Autodesk Inventor part; units mm, degrees
ref_plane "YZ Plane" through (0, 0, 0) normal (1, 0, 0) x (0, 1, 0)
ref_plane "XZ Plane" through (0, 0, 0) normal (0, 1, 0) x (-1, 0, 0)
ref_plane "XY Plane" through (0, 0, 0) normal (0, 0, 1) x (1, 0, 0)
sketch "スケッチ1" plane through (0, 0, 0) normal (1, 0, 0) x (0, 1, 0)
  circle A0 centre (0, 0) radius 17.5
  dimension "d0" = 35
extrude "押し出し1" add sketch "スケッチ1" along normal blind 3
sketch "スケッチ2" plane through (3, 0, 0) normal (1, 0, 0) x (0, 0, -1)
  circle A0 centre (0, 0) radius 13.5
  point P0 (13.5, 0)
  point P1 (6.75, 11.6913)
  point P2 (-6.75, 11.6913)
  point P3 (-13.5, 0)
  point P4 (-6.75, -11.6913)
  point P5 (6.75, -11.6913)
  dimension "d3" = 27
  dimension "d6" = 360
hole "穴1" at (3, 0, -13.5) at (3, 11.6913, -6.75) at (3, 11.6913, 6.75) at (3, 0, 13.5) at (3, -11.6913, 6.75) at (3, -11.6913, -6.75) direction (-1, 0, 0) diameter 3.2 end through all
sketch "スケッチ4" plane through (3, 0, 0) normal (1, 0, 0) x (0, 0, -1)
  circle A0 centre (0, 0) radius 20
  circle A1 centre (0, -20) radius 5
  circle A2 centre (0, 20) radius 5
  circle A3 centre (13.5, 0) radius 1.6
  circle A4 centre (-13.5, 0) radius 1.6
  line L0 (-24.9861, -3.2077) -> (0.509, 28.6357)
  line L1 (1.3172, 26.3548) -> (24.4586, -2.5487)
  line L2 (-28.3137, 7.3638) -> (1.2125, -29.5144)
  line L3 (-0.4955, -28.6189) -> (23.5579, 1.4238)
  circle A5 centre (0, 0) radius 17.5
  point P0 (-3.9031, 23.125)
  point P1 (-13.6609, 10.9375)
  point P2 (-13.6609, -10.9375)
  point P3 (-3.9031, -23.125)
  point P4 (3.9031, -23.125)
  point P5 (13.6609, -10.9375)
  point P6 (13.6609, 10.9375)
  point P7 (3.9031, 23.125)
  dimension "d22" = 40
  dimension "d23" = 10
  dimension "d24" = 10
  dimension "d25" = 13.5
  dimension "d26" = 13.5
extrude "押し出し2" add sketch "スケッチ4" against normal blind 2 contours L1 A5 A2 A0 | A0 A2 L1 | A5 A1 A2 | L3 A1 A0 | A0 A1 A5 L3 | A2 A5 A0 | A0 A2 | A2 A5 | A1 A0 | A0 A1 A5 | A5 A1 | A2 A5 L0 A0 | A0 L0 A2 | A1 L2 A0 | A0 L2 A5 A1
sketch "スケッチ5" plane through (0, 0, 0) normal (-1, 0, 0) x (0, 0, 1)
  circle A0 centre (6.75, -11.6913) radius 1.6
  circle A1 centre (-6.75, -11.6913) radius 1.6
  circle A2 centre (-6.75, 11.6913) radius 1.6
  circle A3 centre (6.75, 11.6913) radius 1.6
  arc A4 (3.9031, 23.125) -> (-3.9031, 23.125) centre (0, 20) ccw
  arc A5 (-3.9031, -23.125) -> (3.9031, -23.125) centre (0, -20) ccw
  point P0 (0, 0)
hole "穴2" at (0, -11.6913, 6.75) at (0, -11.6913, -6.75) at (0, 11.6913, -6.75) at (0, 11.6913, 6.75) at (0, 20, 0) at (0, -20, 0) direction (1, 0, 0) diameter 3.2 depth 5
sketch "スケッチ6" plane through (0, 0, 0) normal (-1, 0, 0) x (0, 0, 1)
  circle A0 centre (0, 0) radius 17.5
extrude "押し出し3" cut sketch "スケッチ6" against normal blind 1
properties part number "endeff_plate2" material "アルミニウム 6061"
Could you check a few things on this model? Use its own coordinates, in mm. Round coordinates to 2 decimals unless told otherwise and drop trailing zeros. Loops run counter-clockwise (first coordinate to the right, second up) from the corner with the lowest first, then second, coordinate; pieces in that order, holes last. Notation, with made-up numbers: (42.25, 14.5) -> (99.25, 14.5) arc R9 cw to (99.25, 24.5) -> close; hole circle Ø6 at (-7, -34). An arc over 180 degrees is marked (long way). Put each result on its own line as item: value.
Q1. I want a section at A-A on z = 0. Write out the boundary of the cut face in (x, y), and give its area (3 significant figures).
Checks:
outline: (1, -25) -> (3, -25) -> (3, -21.6) -> (1, -21.6) -> close; (1, -18.4) -> (3, -18.4) -> (3, 18.4) -> (1, 18.4) -> close; (1, 21.6) -> (3, 21.6) -> (3, 25) -> (1, 25) -> close
area: 87.2 mm2
Q2. For pin 1 Ø2.5 at (y, z) = (-11.69, 6.75) entering from +X; pin 2 Ø1 at (x, y) = (1.5, 14) entering from -Z, each with a flat end and sliding along its axis, tell me the tip position at first contact or that it passes through.
Checks:
pin 1: through
pin 2: z = -11.61
Q3. Please list where these lines run through material, in increasing order: line 1 (Z direction, x = 2.15, y = 0); line 2 (Z direction, x = 1.85, y = 13); line 3 (Y direction, x = 1.4, z = -5.5). Write a range as from..to.
Checks:
line 1: -17.5..-15.1, -11.9..11.9, 15.1..17.5
line 2: -12.01..-7.67, -5.83..5.83, 7.67..12.01
line 3: -21.13..-12.69, -10.69..10.69, 12.69..21.13
Q4. I want a section at D-D on z = -12.5. Write out the boundary of the cut face in (x, y).
Checks:
outline: (1, -12.39) -> (3, -12.39) -> (3, -1.25) -> (1, -1.25) -> close; (1, 1.25) -> (3, 1.25) -> (3, 12.39) -> (1, 12.39) -> close
Q5. I want a section at B-B on y = 0. Write out the boundary of the cut face in (x, z), and give its area (3 significant figures).
Checks:
outline: (1, -17.5) -> (3, -17.5) -> (3, -15.1) -> (1, -15.1) -> close; (1, -11.9) -> (3, -11.9) -> (3, 11.9) -> (1, 11.9) -> close; (1, 15.1) -> (3, 15.1) -> (3, 17.5) -> (1, 17.5) -> close
area: 57.2 mm2
Q6. I want a section at C-C on y = -20. Write out the boundary of the cut face in (x, z).
Checks:
outline: (1, -6.41) -> (3, -6.41) -> (3, -1.6) -> (1, -1.6) -> close; (1, 1.6) -> (3, 1.6) -> (3, 6.41) -> (1, 6.41) -> close
Q7. Thinking about a two-plate mould opening in Z: for faces 1 (the cylindrical face through (2, 25, 0)), 2 (the flat face through (2.01, 17.12, -8.71)), 3 (the cylindrical face through (1.99, -0.07, -11.9)), which applies, pulls with the +Z half, pulls with the -Z half, needs draft (parallel to the pull), parting line crosses it, or undercut?
Checks:
face 1: parting line crosses it
face 2: pulls with the -Z half
face 3: undercut
